Part model, mm, in its own coordinate system. A direction names the side the tool comes from. Round coordinates to 2 decimals unless told otherwise and drop trailing zeros. Write each loop counter-clockwise with the first axis right and the second up, starting at its lowest first coordinate (ties: lowest second). Pieces come first, ordered by that corner, then holes.
1) Saw through at A-A on z = -4.5. Write the cut outline in (x, y) (1 decimal).
2) Saw through at B-B on y = -24.5. Write the cut outline in (x, z) (1 decimal), and give its area (3 significant figures).
3) Saw through at D-D on x = 89. Write the cut outline in (y, z) (3 decimals).
4) Which spindle directions (+Z, -Z, +X, -X, +Y, -Y) get a long thin tool onto all of the face, cutting with end or side? Do faces 1 (the flat face through (203.2, -5, -26)), 2 (the flat face through (102, -98.425, -6)), 3 (the flat face through (96.838, -43, -29)), 4 (the flat face through (106.362, -43, -30)). Say none if no direction does.
5) Drill centre lines: L1, parallel to Z at x = 155.5, y = -85.5 (3 decimals); L2, parallel to Y at x = 56, z = -23 (3 decimals); L3, parallel to X at y = -7, z = -76.5. Where is each one in solid material? Low to high.
6) Saw through at C-C on x = 61. Write the cut outline in (y, z) (3 decimals), and give its area (3 significant figures).
7) Flat gauge pins, fed straight in: pin 1 (3 mm diameter, centred on y = -2.5, z = -18.5, fed in from -X); pin 2 (5 mm diameter, centred on x = 14, y = -24.5, fed in from -Z); pin 3 (23 mm diameter, centred on y = -63, z = -25.5, fed in from -X); pin 4 (12 mm diameter, centred on x = 76, z = -23, fed in from +Y). Where does each tip first touch, or does it go through?
```python
from build123d import *

# Parameters (mm, degrees)
F1_DEPTH = 9.525
F3_DEPTH = 88.9
F5_DEPTH = 9.525
F7_DEPTH = 9.525


# Not quite as in the source:
# - a length typed as a fraction of an inch, garbled in the dataset ("3 / 203.2 mm" for 3/8 in), is restored


with BuildPart() as f1:
    # F0 (on Front) → F1 (new body)
    with BuildSketch(Plane.XZ):
        with BuildLine():
            Line((203.2, 0), (0, 0))
            Line((0, 0), (0, -50.8))
            ThreePointArc((0, -50.8), (17.9605122421, -58.2394877579), (25.4, -76.2))
            Line((25.4, -76.2), (76.2, -76.2))
            ThreePointArc((76.2, -76.2), (101.6, -101.6), (127, -76.2))
            Line((127, -76.2), (177.8, -76.2))
            ThreePointArc((177.8, -76.2), (185.2394877579, -58.2394877579), (203.2, -50.8))
            Line((203.2, -50.8), (203.2, 0))
        make_face()
    extrude(amount=F1_DEPTH)

    # F2 (on face) → F3 (join)
    with BuildSketch(Plane.XZ.offset(9.525)):
        Polygon((96.8375, 0), (96.8375, -76.2), (101.6, -76.2), (106.3625, -76.2), (106.3625, 0), align=None)
    extrude(amount=F3_DEPTH)

    # F4 (on face) → F5 (cut)
    with BuildSketch(Plane.YZ.offset(106.3625)):
        with BuildLine():
            Line((-98.425, -76.2), (-28.575, -76.2))
            ThreePointArc((-28.575, -76.2), (-52.4826849385, -32.3309534324), (-98.425, -12.7))
            Line((-98.425, -12.7), (-98.425, -76.2))
        make_face()
    extrude(amount=-F5_DEPTH, mode=Mode.SUBTRACT)

    # F6 (on face) → F7 (join)
    with BuildSketch(Plane.XY):
        with BuildLine():
            Line((0, -9.525), (0, 0))
            Line((0, 0), (-12.7, 0))
            Line((-12.7, 0), (-12.7, -88.9))
            ThreePointArc((-12.7, -88.9), (-5.2605122421, -106.8605122421), (12.7, -114.3))
            Line((12.7, -114.3), (190.5, -114.3))
            ThreePointArc((190.5, -114.3), (208.4605122421, -106.8605122421), (215.9, -88.9))
            Line((215.9, -88.9), (215.9, 0))
            Line((215.9, 0), (203.2, 0))
            Line((203.2, 0), (203.2, -9.525))
            Line((203.2, -9.525), (106.3625, -9.525))
            Line((106.3625, -9.525), (106.3625, -98.425))
            Line((106.3625, -98.425), (96.8375, -98.425))
            Line((96.8375, -98.425), (96.8375, -9.525))
            Line((96.8375, -9.525), (0, -9.525))
        make_face()
        Polygon((203.2, 0), (0, 0), (0, -9.525), (96.8375, -9.525), (96.8375, -98.425), (106.3625, -98.425), (106.3625, -9.525), (203.2, -9.525), align=None)
    extrude(amount=F7_DEPTH)


solid = f1.part
```
Completed:
1. outline: (0, -9.5) - (96.8, -9.5) - (96.8, -98.4) - (106.4, -98.4) - (106.4, -9.5) - (203.2, -9.5) - (203.2, 0) - (0, 0) - close
2. outline: (-12.7, 0) - (96.8, 0) - (96.8, -76.2) - (106.4, -76.2) - (106.4, 0) - (215.9, 0) - (215.9, 9.5) - (-12.7, 9.5) - close
2. area: 2,900 mm2
3. outline: (-114.3, 0) - (-9.525, 0) - (-9.525, -98.254) - (0, -98.254) - (0, 9.525) - (-114.3, 9.525) - close
4. face 1: -Z, +X, +Y, -Y
4. face 2: -Z, +X, -X, -Y
4. face 3: -Z, -X, -Y
4. face 4: -Z, +X, -Y
5. L1: z = 0 to 9.525
5. L2: y = -9.525 to 0
5. L3: x = 76.2 to 127
6. outline: (-114.3, 0) - (-9.525, 0) - (-9.525, -76.2) - (0, -76.2) - (0, 9.525) - (-114.3, 9.525) - close
6. area: 1,810 mm2
7. pin 1: stops at x = 0
7. pin 2: stops at z = 0
7. pin 3: stops at x = 96.84
7. pin 4: stops at y = 0
